CAD build for the part. Positions are in the model's coordinates, mm. Face numbers are marked on the shaded views. A direction names the side the tool comes from. Give positions to 0.01 mm unless a question says otherwise; leave off trailing zeros. Write each loop counter-clockwise with the first axis right and the second up, starting at its lowest first coordinate (ties: lowest second). Pieces come first, ordered by that corner, then holes. Notation, with made-up numbers: (30, 84.5) - (71, 84.5) arc R18 ccw to (71, 92.5) - close; hole circle Ø11 at (70, 54). An arc over 180 degrees is marked (long way). Answer as a JSON object with one key per item and string values.
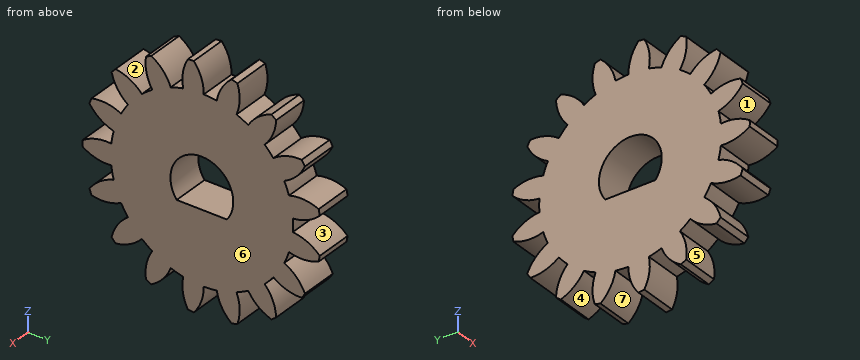
from build123d import *

# Parameters (mm, degrees)
BASPROSKE_W     = 3
BASPROSKE_H     = 9.5
TOOTHCUT_DEPTH  = 14.765899898
TEETHCUTS_COUNT = 17
TEETHCUTS_ANGLE = 338.823529412
BORSKE_R        = 2.5
BORE_DEPTH      = 50.0000508
EXTRUDE_1_DEPTH = 3


with BuildPart() as part:
    # BasProSke → Base-Revolve (revolve)
    with BuildSketch(Plane(origin=(0, 0, 0), x_dir=(1, 0, 0), z_dir=(0, 1, 0)), mode=Mode.PRIVATE) as base_revolve_sk:
        with Locations((1.5, 4.75)):
            Rectangle(BASPROSKE_W, BASPROSKE_H)
    revolve(base_revolve_sk.sketch.rotate(Axis((-10, 0, 0), (1, 0, 0)), 180), axis=Axis((-10, 0, 0), (1, 0, 0)))

    # TooCutSke → ToothCut (cut, through all)
    with BuildSketch(Plane(origin=(0, 0, 0), x_dir=(0, 0, -1), z_dir=(1, 0, 0))):
        with BuildLine():
            ThreePointArc((0.516861231, 7.23055015), (0, 7.249), (-0.516861231, 7.23055015))
            ThreePointArc((-0.516861231, 7.23055015), (-0.827352654, 8.408398361), (-1.533069197, 9.401220346))
            ThreePointArc((-1.533069197, 9.401220346), (0, 9.5254), (1.533069197, 9.401220346))
            ThreePointArc((1.533069197, 9.401220346), (0.827352654, 8.408398361), (0.516861231, 7.23055015))
        make_face()
    toothcut = extrude(amount=TOOTHCUT_DEPTH, mode=Mode.SUBTRACT)

    # TeethCuts: ToothCut ×17 about axis
    teethcuts_axis = Axis((-10, 0, 0), (1, 0, 0))
    for i in range(1, TEETHCUTS_COUNT):
        add(toothcut.rotate(teethcuts_axis, i * TEETHCUTS_ANGLE / (TEETHCUTS_COUNT - 1)), mode=Mode.SUBTRACT)

    # BorSke → Bore (cut, symmetric)
    with BuildSketch(Plane(origin=(0, 0, 0), x_dir=(0, 0, -1), z_dir=(1, 0, 0))):
        with Locations(Location((0, 0, 0), (0, 0, 180))):
            Circle(BORSKE_R)
    extrude(amount=BORE_DEPTH, both=True, mode=Mode.SUBTRACT)

    # 草图1 → 凸台-拉伸1 (add)
    with BuildSketch(Plane(origin=(3, 0, 0), x_dir=(0, 0, -1), z_dir=(1, 0, 0))):
        with BuildLine():
            Line((1.5, 2), (1.5, -2))
            ThreePointArc((1.5, -2), (2.5, 0), (1.5, 2))
        make_face()
    extrude(amount=-EXTRUDE_1_DEPTH)


solid = part.part
(1) Pull direction Y, two halves, no side cores. Call the marked faces 1, 2, 3 and 4: pulls with the +Y half, pulls with the -Y half, needs draft (parallel to the pull), parting line crosses it, or undercut.
Answer key:
{"face 1": "pulls with the -Y half", "face 2": "undercut", "face 3": "pulls with the +Y half", "face 4": "undercut"}
(2) Probe L1, parallel to Y at x = 2.15, z = 0; L2, parallel to Y at x = 1.8, z = 8.5; L3, parallel to Z at x = 2.85, y = -7.5. List the from-to ranges inside material, lowest first. Write a range as [from, to].
Answer key:
{"L1": "y = [-9.5, -2.5], [2.5, 7.25]", "L2": "y = [-4.24, -3.84], [-1.47, -0.07], [1.73, 2.97]", "L3": "z = [-3.71, -2.01], [-0.84, 0.84], [2.01, 3.71]"}
(3) Saw through at A-A, the plane z = 0. Give the cut face in (x, y).
Answer key:
{"outline": "(0, -9.5) - (3, -9.5) - (3, -2.5) - (0, -2.5) - close; (0, 2.5) - (3, 2.5) - (3, 7.25) - (0, 7.25) - close"}
(4) 3-axis set-ups, long thin cutter, end or side, ignore diameter. For the marked faces 5, 6 and 7: which of +Z, -Z, +X, -X, +Y, -Y reach the whole face in a straight line?
Answer key:
{"face 5": "+X, -X", "face 6": "+Z, -Z, +X, +Y, -Y", "face 7": "-Z, +X, -X"}
(5) Saw through at B-B, the plane y = -8.5. Give the cut face in (x, z).
Answer key:
{"outline": "(0, -3.71) - (3, -3.71) - (3, -2.68) - (0, -2.68) - close; (0, -0.71) - (3, -0.71) - (3, 0.71) - (0, 0.71) - close; (0, 2.68) - (3, 2.68) - (3, 3.71) - (0, 3.71) - close"}
(6) Flat gauge pins, fed straight in: P1, Ø1.5, axis at x = 2, y = -3.5, coming from the -Z side; P2, Ø1.5, axis at x = 2, y = -0.5, coming from the +Z side. Where does each tip first touch, or does it go through?
Answer key:
{"P1": "stops at z = -8.61", "P2": "stops at z = 9.48"}
